Input: part model. Units: mm. Frame: model coordinates. A direction names the side the tool comes from. Coordinates: 2 decimals unless noted, no trailing zeros. Loops run counter-clockwise (first coordinate to the right, second up) from the corner with the lowest first, then second, coordinate; pieces in that order, holes last. Notation, with made-up numbers: (-14, 19) -> (36, 19) arc R25 ccw to (36, 58) -> close; hole circle Ø3 at (38, 14.5). An arc over 180 degrees is marked (long way). Answer as a JSON object with one key per item and string values.
Autodesk Inventor part; units mm, degrees
ref_plane "YZ Plane" through (0, 0, 0) normal (1, 0, 0) x (0, 1, 0)
ref_plane "XZ Plane" through (0, 0, 0) normal (0, 1, 0) x (-1, 0, 0)
ref_plane "XY Plane" through (0, 0, 0) normal (0, 0, 1) x (1, 0, 0)
sketch "Sketch1" plane through (0, 0, 0) normal (0, 1, 0) x (-1, 0, 0)
  line L0 (-37.4, -24.6) -> (-287.4, -24.6)
  line L1 (-287.4, -24.6) -> (-287.4, 175.4)
  line L2 (-287.4, 175.4) -> (-37.4, 175.4)
  line L3 (-37.4, 175.4) -> (-37.4, -24.6)
  line L4 (-37.4, -7.6) -> (-270.4, -7.6)
  line L5 (-270.4, -7.6) -> (-270.4, 158.4)
  line L6 (-270.4, 158.4) -> (-37.4, 158.4)
  line L7 (-244.2, 150.4) -> (-265.4, 150.4)
  line L8 (-265.4, 0.4) -> (-244.2, 0.4)
  line L9 (-265.4, 0.4) -> (-244.2, 0.4)
  point P0 (0, 0)
  dimension "d0" = 250
  dimension "d1" = 200
  dimension "offset_claw_nuts" = 17
  dimension "d3" = 17
  dimension "d4" = 17
  dimension "d5" = 8
  dimension "d6" = 8
  dimension "d7" = 5
extrude "Extrusion1" add sketch "Sketch1" along normal blind 25 and the other way blind 7 contours L0 L1 L2 L3 L6 L5 L4
sketch "Sketch2" plane through (0, -7, 0) normal (0, -1, 0) x (1, 0, 0)
  line L0 (287.4, -24.6) -> (287.4, 175.4)
  line L1 (287.4, 175.4) -> (37.4, 175.4)
  line L2 (37.4, 175.4) -> (37.4, 158.4)
  line L3 (37.4, 158.4) -> (270.4, 158.4)
  line L4 (270.4, 158.4) -> (270.4, -7.6)
  line L5 (270.4, -7.6) -> (37.4, -7.6)
  line L6 (37.4, -7.6) -> (37.4, -24.6)
  line L7 (37.4, -24.6) -> (287.4, -24.6)
  line L8 (37.4, -24.6) -> (37.4, -24.6)
  line L9 (37.4, -24.6) -> (37.4, 175.4)
  line L10 (37.4, 175.4) -> (37.4, 175.4)
  line L11 (37.4, 175.4) -> (37.4, -24.6)
  point P0 (0, 0)
  point P1 (37.4, 158.4)
  point P2 (37.4, -7.6)
extrude "Extrusion2" add sketch "Sketch2" against normal blind 3 contours L9 L3 L4 L5
sketch "Sketch3" plane through (37.4, -7, 175.4) normal (-1, 0, 0) x (0, 0, 1)
  line L0 (0, 0) -> (0, 32)
  line L1 (-17, 32) -> (0, 32)
  line L2 (-17, 3) -> (-17, 32)
  line L3 (-183, 3) -> (-17, 3)
  line L4 (-183, 3) -> (-183, 32)
  line L5 (-200, 32) -> (-183, 32)
  line L6 (-200, 0) -> (-200, 32)
  line L7 (0, 0) -> (-200, 0)
  line L8 (-183, 32) -> (-183, 32)
  line L9 (-183, 32) -> (-183, 32) construction
  line L10 (-183, 32) -> (-183, 9)
  line L11 (0, 32) -> (-200, 32)
  line L12 (-183, 9) -> (-17, 9)
  line L13 (-17, 9) -> (-17, 32)
  line L14 (-17, 32) -> (-17, 32)
  point P0 (-175.4, 7)
  point P1 (-75, 9)
  point P2 (-17, 9)
  dimension "d14" = 45
  dimension "d16" = 135
  dimension "d17" = 0
  dimension "d18" = 6
  dimension "d19" = 0
  dimension "d20" = 125
  dimension "d21" = 75
extrude "Extrusion3" add sketch "Sketch3" against normal blind 2.5 contours L2 L3 L4 L12
sketch "Sketch4" plane through (0, -4, 0) normal (0, 1, 0) x (1, 0, 0)
  line L0 (39.9, 7.6) -> (39.9, -158.4)
  line L1 (270.4, -158.4) -> (39.9, -158.4)
  line L2 (270.4, 7.6) -> (270.4, -158.4)
  line L3 (39.9, 7.6) -> (270.4, 7.6)
  line L4 (270.4, 7.6) -> (270.4, -158.4)
  line L5 (270.4, -158.4) -> (39.9, -158.4)
  line L6 (270.4, 7.6) -> (69.9, 7.6)
  line L7 (69.9, 7.6) -> (69.9, -158.4)
  line L8 (69.9, -158.4) -> (270.4, -158.4)
  line L9 (270.4, -158.4) -> (270.4, 7.6)
  point P0 (0, 0)
  point P1 (69.9, 7.6)
  point P2 (69.9, -158.4)
  dimension "d26" = 30
extrude "Extrusion4" add sketch "Sketch4" along normal up to surface (6 mm away) contours L3 L2 L1 L7
sketch "Sketch6" plane through (39.9, -7, 175.4) normal (1, 0, 0) x (0, 0, -1)
  line L0 (17, 3) -> (17, 9)
  line L1 (183, 3) -> (17, 3)
  line L2 (183, 9) -> (183, 3)
  line L3 (183, 9) -> (17, 9)
  circle A0 centre (20, 6) radius 3
  circle A1 centre (42.8571, 6) radius 3
  circle A2 centre (65.7143, 6) radius 3
  circle A3 centre (88.5714, 6) radius 3
  circle A4 centre (111.4286, 6) radius 3
  circle A5 centre (134.2857, 6) radius 3
  circle A6 centre (157.1429, 6) radius 3
  circle A7 centre (180, 6) radius 3
  point P0 (175.4, 7)
  dimension "d29" = 6
  dimension "d30" = 6
  dimension "d31" = 6
  dimension "d32" = 6
  dimension "d33" = 6
  dimension "d34" = 6
  dimension "d35" = 6
  dimension "d36" = 6
  dimension "d37" = 22.8571
  dimension "d38" = 22.8571
  dimension "d39" = 22.8571
  dimension "d40" = 22.8571
  dimension "d41" = 22.8571
  dimension "d42" = 22.8571
  dimension "d43" = 22.8571
hole "Hole1" at (39.9, -1, -4.6) at (39.9, -1, 18.2571) at (39.9, -1, 41.1143) at (39.9, -1, 63.9714) at (39.9, -1, 86.8286) at (39.9, -1, 132.5429) at (39.9, -1, 155.4) at (39.9, -1, 109.6857) direction (-1, 0, 0) diameter 3.6 end through all
sketch "Sketch7" plane through (0, 25, 0) normal (0, 1, 0) x (1, 0, 0)
  line L0 (287.4, -175.4) -> (287.4, 24.6)
  line L1 (287.4, 24.6) -> (37.4, 24.6)
  line L2 (37.4, 24.6) -> (37.4, 7.6)
  line L3 (37.4, 7.6) -> (270.4, 7.6)
  line L4 (270.4, 7.6) -> (270.4, -158.4)
  line L5 (270.4, -158.4) -> (37.4, -158.4)
  line L6 (37.4, -158.4) -> (37.4, -175.4)
  line L7 (37.4, -175.4) -> (287.4, -175.4)
  circle A0 centre (278.9, 16.1) radius 8.5
  circle A1 centre (278.9, -166.9) radius 8.5
  circle A2 centre (201.2333, 16.1) radius 8.5
  circle A3 centre (201.2333, -166.9) radius 8.5
  circle A4 centre (278.9, -75.4) radius 8.5
  circle A5 centre (123.5667, 16.1) radius 8.5
  circle A6 centre (123.5667, -166.9) radius 8.5
  circle A7 centre (45.9, 16.1) radius 8.5 construction
  circle A8 centre (45.9, -166.9) radius 8.5 construction
  point P0 (0, 0)
  dimension "d51" = 17
  dimension "d52" = 17
  dimension "d55" = 17
  dimension "d56" = 17
  dimension "d57" = 17
  dimension "d58" = 17
  dimension "d59" = 17
  dimension "d60" = 91.5
  dimension "d61" = 91.5
  dimension "d62" = 77.6667
  dimension "d63" = 77.6667
  dimension "d64" = 17
  dimension "d65" = 17
  dimension "d66" = 8.5
  dimension "d67" = 8.5
  dimension "d68" = 8.5
  dimension "d69" = 8.5
  dimension "d70" = 8.5
  dimension "d71" = 77.6667
  dimension "d72" = 77.6667
  dimension "d73" = 77.6667
  dimension "d74" = 77.6667
  dimension "d75" = 8.5
hole "Hole2" at (123.5667, 25, -16.1) at (278.9, 25, -16.1) at (278.9, 25, 75.4) at (278.9, 25, 166.9) at (201.2333, 25, 166.9) at (201.2333, 25, -16.1) at (123.5667, 25, 166.9) direction (0, -1, 0) diameter 1 end through all
sketch "Sketch8" plane through (0, 25, 0) normal (0, 1, 0) x (1, 0, 0)
  circle A0 centre (201.2333, 16.1) radius 0.5
  circle A1 centre (278.9, -166.9) radius 0.5
  circle A2 centre (278.9, 16.1) radius 0.5
  circle A3 centre (123.5667, 16.1) radius 0.5
  circle A4 centre (278.9, -75.4) radius 0.5
  circle A5 centre (201.2333, -166.9) radius 0.5
  circle A6 centre (123.5667, -166.9) radius 0.5
  line L0 (287.4, -175.4) -> (287.4, 24.6)
  line L1 (287.4, 24.6) -> (37.4, 24.6)
  line L2 (37.4, 24.6) -> (37.4, 7.6)
  line L3 (37.4, 7.6) -> (270.4, 7.6)
  line L4 (270.4, 7.6) -> (270.4, -158.4)
  line L5 (270.4, -158.4) -> (37.4, -158.4)
  line L6 (37.4, -158.4) -> (37.4, -175.4)
  line L7 (37.4, -175.4) -> (287.4, -175.4)
  circle A7 centre (65.9, 16.1) radius 8.5
  circle A8 centre (65.9, -166.9) radius 8.5
  circle A9 centre (278.9, -29.65) radius 8.5
  circle A10 centre (278.9, -121.15) radius 8.5
  circle A11 centre (261.9, 16.1) radius 8.5
  circle A12 centre (261.9, -166.9) radius 8.5
  circle A13 centre (162.4, 16.1) radius 8.5
  circle A14 centre (162.4, -166.9) radius 8.5
  line L8 (37.4, 24.6) -> (287.4, 24.6)
  line L9 (270.4, 7.6) -> (270.4, -158.4)
  line L10 (270.4, 24.6) -> (270.4, 7.6)
  line L11 (270.4, -158.4) -> (270.4, -175.4)
  point P0 (0, 0)
  dimension "d83" = 17
  dimension "d84" = 17
  dimension "d85" = 45.75
  dimension "d86" = 45.75
  dimension "d87" = 45.75
  dimension "d88" = 38.8333
  dimension "d89" = 38.8333
  dimension "d90" = 38.8333
  dimension "d91" = 38.8333
  dimension "d92" = 28.5
  dimension "d93" = 0
hole "Hole3" at (261.9, 25, -16.1) at (278.9, 25, 29.65) at (278.9, 25, 121.15) at (261.9, 25, 166.9) at (162.4, 25, -16.1) at (65.9, 25, -16.1) at (65.9, 25, 166.9) at (162.4, 25, 166.9) direction (0, -1, 0) diameter 3 end through all
equation "\"d3\" = offset_claw_nuts"
equation "\"d4\" = offset_claw_nuts"
equation "\"d6\" = d5"
equation "\"d37\" = d43"
equation "\"d38\" = d43"
equation "\"d39\" = d43"
equation "\"d40\" = d43"
equation "\"d41\" = d43"
equation "\"d42\" = d43"
equation "\"d60\" = d61"
equation "\"d62\" = d71"
equation "\"d63\" = d71"
equation "\"d66\" = 0.5 * d58"
equation "\"d67\" = 0.5 * d64"
equation "\"d68\" = 0.5 * d64"
equation "\"d69\" = 0.5 * d65"
equation "\"d70\" = 0.5 * d65"
equation "\"d72\" = d74"
equation "\"d73\" = d74"
properties part number "case0"
1. Section query A-A (z = 4.5). Return loops of the section in (x, y), plus the area to 3 significant figures.
Reply:
{"outline": "(37.4, -7) -> (287.4, -7) -> (287.4, 25) -> (270.4, 25) -> (270.4, 2) -> (69.9, 2) -> (69.9, -4) -> (39.9, -4) -> (39.9, 2) -> (37.4, 2) -> close", "area": "2,460 mm2"}
2. Section query C-C (y = 5). Count the separate pieces of the cut face and the enclosed holes in it, plus the area to 3 significant figures.
Reply:
{"separate pieces": "1", "enclosed holes": "15", "area": "11,300 mm2"}
3. Mould query, pull axis Z, two halves, no side actions, for faces 4 (the face through (39.9, -1, 74)), 5 (the face through (164, 9, 175.4)), 6 (the face through (274, 25, 68)). Classes: pulls with the +Z half, pulls with the -Z half, needs draft (parallel to the pull), parting line crosses it, or undercut.
Reply:
{"face 4": "undercut", "face 5": "pulls with the +Z half", "face 6": "needs draft"}
4. Line query: line 1 along Z through (x, y) = (65.9, 7); line 2 along Z through (x, y) = (278.9, 5.5); line 3 along X through (y, z) = (1, 154). Output: solid intervals per line, ascending.
Reply:
{"line 1": "z = -24.6 to -17.6, -14.6 to -7.6, 158.4 to 165.4, 168.4 to 175.4", "line 2": "z = -24.6 to -16.6, -15.6 to 28.15, 31.15 to 74.9, 75.9 to 119.65, 122.65 to 166.4, 167.4 to 175.4", "line 3": "x = 37.4 to 39.9, 69.9 to 287.4"}
5. Section query B-B (x = 154). Return loops of the section in (y, z).
Reply:
{"outline": "(-7, -24.6) -> (25, -24.6) -> (25, -7.6) -> (2, -7.6) -> (2, 158.4) -> (25, 158.4) -> (25, 175.4) -> (-7, 175.4) -> close"}
6. Pin query (flat end, axial travel): P1, Ø2.5, axis at x = 261.9, z = 166.9, coming from the +Y side; P2, Ø12, axis at x = 131, z = 108.5, coming from the +Y side; P3, Ø1, axis at y = 7, z = 14.5, coming from the -X side. Return the tip coordinate at first contact, or that it passes through.
Reply:
{"P1": "passes through", "P2": "stops at y = 2", "P3": "stops at x = 270.4"}
7. Access query for faces 1 (the face through (270.4, 13, 74)), 2 (the face through (161, -7, 77)), 3 (the face through (55, -4, 77)). Directions: +Z, -Z, +X, -X, +Y, -Y. A direction counts if a zero-diameter tool reaches every point of the face in a straight line with its end or side. Return the directions, or none.
Reply:
{"face 1": "-X, +Y", "face 2": "+Z, -Z, +X, -X, -Y", "face 3": "+Y"}
